The listing builds one solid part. Answer for the finished solid, in the listing's coordinates (mm). A direction names the side the tool comes from. Give positions to 0.01 mm unless a question says otherwise; leave off trailing zeros. Order: outer loops, then holes, each group sorted by start corner. A loop starts at its lowest first (then second) coordinate and runs counter-clockwise, first axis right, second up. Notation, with made-up numbers: (-32, -14.5) -> (-24, -14.5) arc R27 ccw to (-24, 12.5) -> close; hole circle Ø9 at (8, -8.75). An arc over 180 degrees is marked (long way). Write item = value, one per line. Start each with the question number.
```python
from build123d import *

# Parameters (mm, degrees)
CROQUIS1_W              = 3
CROQUIS1_H              = 57
SALIENTE_EXTRUIR1_DEPTH = 17.5
CROQUIS2_R              = 3
SALIENTE_EXTRUIR2_DEPTH = 25
CROQUIS3_R              = 4.7625
SALIENTE_EXTRUIR3_DEPTH = 55


with BuildPart() as part:
    # Croquis1 → Saliente-Extruir1 (new, symmetric)
    with BuildSketch(Plane.XY):
        with Locations((1.5, 28.5)):
            Rectangle(CROQUIS1_W, CROQUIS1_H)
        Polygon((3, 0), (0, 0), (0, -3), (63, -3), (63, 0), align=None)
    extrude(amount=SALIENTE_EXTRUIR1_DEPTH, both=True)

    # Croquis2 → Saliente-Extruir2 (add)
    with BuildSketch(Plane(origin=(3, 0, 0), x_dir=(0, 0, -1), z_dir=(1, 0, 0))):
        with Locations(Location((0, 25, 0), (0, 0, 180))):
            Circle(CROQUIS2_R)
    extrude(amount=SALIENTE_EXTRUIR2_DEPTH)

    # Croquis3 → Saliente-Extruir3 (add)
    with BuildSketch(Plane(origin=(0, 0, 0), x_dir=(1, 0, 0), z_dir=(0, 1, 0))):
        with Locations(Location((33, 0, 0), (0, 0, 270))):
            Circle(CROQUIS3_R)
    extrude(amount=SALIENTE_EXTRUIR3_DEPTH)


solid = part.part
```
Item 1: Which of the six approach directions +Z, -Z, +X, -X, +Y, -Y give full straight-line access (tool end or side, diameter ignored) to faces 1 (the cylindrical face through (15.32, 27.93, -0.65)), 2 (the flat face through (28, 25, 0)), 3 (the flat face through (33, 55, 0)), 4 (the cylindrical face through (37.72, 27.12, -0.62))?
Item 2: A cutting plane is placed at A-A, the plane y = 25. Write down the section's boundary in (x, z) (1 decimal).
Item 3: The mould has two halves that part along X. Classify faces 5 (the flat face through (0, 27, 0)), 6 (the flat face through (63, -2, 0)), 7 (the flat face through (40, 0, 0)), 8 (the flat face through (1, 57, 0)): +X half, -X half, draft (parallel to the pull), parting line (faces both ways), or undercut.
Item 4: Consider L1, parallel to Y at x = 5, z = -4; L2, parallel to X at y = 7, z = -15; L3, parallel to Y at x = 13.5, z = 0.5. Determine where each line is inside the solid, lowest interval first. Write a range as from..to.
Item 5: Flat-ended cylindrical pins translate along their axes: pin 1 (10.5 mm diameter, centred on y = 31, z = -2.5, fed in from +X); pin 2 (10 mm diameter, centred on y = 15, z = -5.5, fed in from +X); pin 3 (17.5 mm diameter, centred on x = 38, z = -7, fed in from +Y). Find the tip coordinate at first contact, or state that the pin passes through.
Item 6: A cutting plane is placed at B-B, the plane x = 19. Write down the section's boundary in (y, z), plus the area to 3 significant figures.
Item 7: A cutting plane is placed at D-D, the plane z = 0. Write down the section's boundary in (x, y).
Item 8: A cutting plane is placed at C-C, the plane x = 33. Write down the section's boundary in (y, z), plus the area to 3 significant figures.
Check values:
q1.face_1 = none
q1.face_2 = +Z, -Z, +Y
q1.face_3 = +Z, -Z, +X, +Y
q1.face_4 = +Y
q2.outline = (0, -17.5) -> (3, -17.5) -> (3, -3) -> (28, -3) -> (28, 3) -> (3, 3) -> (3, 17.5) -> (0, 17.5) -> close; circle Ø9.5 at (33, 0)
q3.face_5 = -X half
q3.face_6 = +X half
q3.face_7 = undercut
q3.face_8 = draft
q4.L1 = -3..0
q4.L2 = 0..3
q4.L3 = -3..0, 22.04..27.96
q5.pin_1 = 37.76
q5.pin_2 = 37.74
q5.pin_3 = 55
q6.outline = (-3, -17.5) -> (0, -17.5) -> (0, 17.5) -> (-3, 17.5) -> close; circle Ø6 at (25, 0)
q6.area = 133 mm^2
q7.outline = (0, -3) -> (63, -3) -> (63, 0) -> (37.76, 0) -> (37.76, 55) -> (28.24, 55) -> (28.24, 0) -> (3, 0) -> (3, 22) -> (28, 22) -> (28, 28) -> (3, 28) -> (3, 57) -> (0, 57) -> close
q8.outline = (-3, -17.5) -> (0, -17.5) -> (0, -4.76) -> (55, -4.76) -> (55, 4.76) -> (0, 4.76) -> (0, 17.5) -> (-3, 17.5) -> close
q8.area = 629 mm^2
